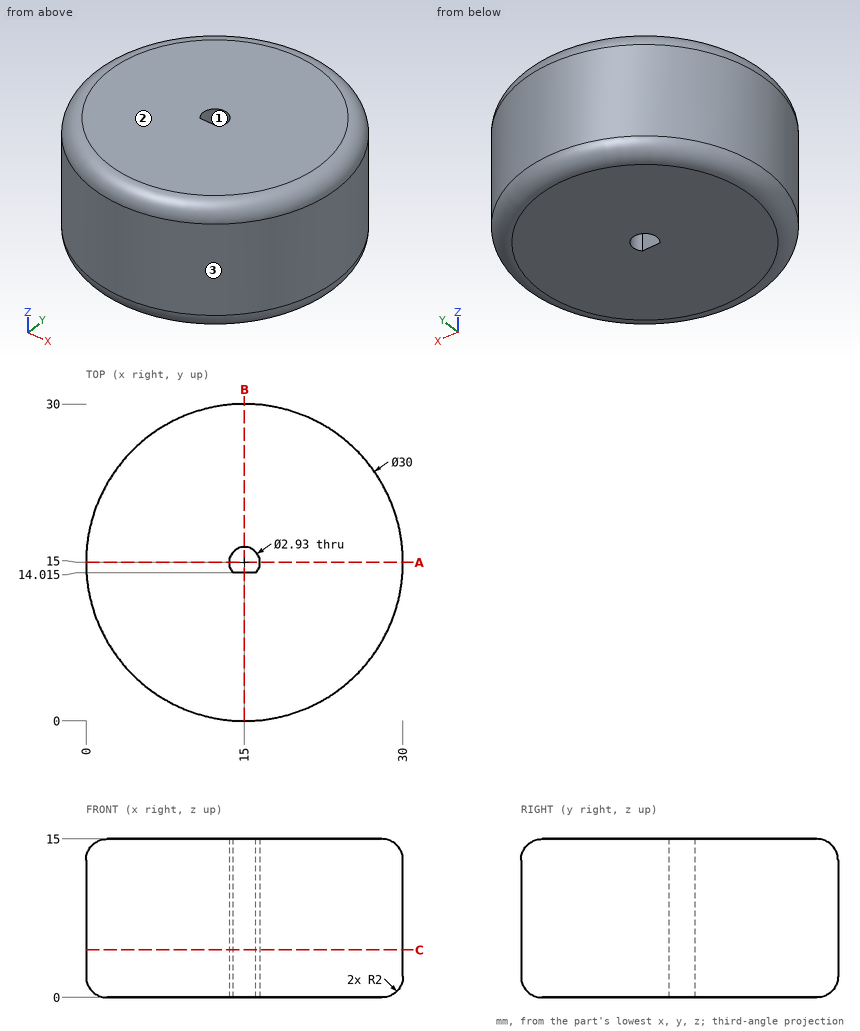
Study the drawing (mm; zero at the part's minimum x, y, z) and answer. Give positions to 0.01 mm unless a question says otherwise; leave off trailing zeros. Loops run counter-clockwise (first coordinate to the right, second up) from the corner with the lowest first, then second, coordinate; pieces in that order, holes last. Notation, with made-up numbers: (31.5, 75.5) - (41.5, 75.5) arc R27 ccw to (41.5, 99.5) - close; hole circle Ø10 at (-34.5, 9.25). An arc over 180 degrees is marked (long way). Use CSV: the item, a comma, the result in double quotes. Start each with the question number.
(1) Find section B-B, the plane x = 15. Determine the outline of the cut face in (y, z) (3 decimals), plus the area to 3 significant figures.
(2) Each of these flat-tipped pins is pushed along its axis until it touches: pin 1 (6 mm diameter, centred on y = 19, z = 11, fed in from -X); pin 2 (1 mm diameter, centred on y = 13, z = 9, fed in from +X); pin 3 (1.5 mm diameter, centred on y = 9.5, z = 11, fed in from +X); pin 4 (1.8 mm diameter, centred on x = 15, y = 15, fed in from -Z). Where does it stop, or does it pass through?
(3) Find section C-C, the plane z = 4.5. Determine the outline of the cut face in (x, y) (1 decimal), plus the area to 3 significant figures.
(4) Find section A-A, the plane y = 15. Determine the outline of the cut face in (x, z) (3 decimals), plus the area to 3 significant figures.
(5) Determine the mould class of the marked faces 1, 2 and 3 for opening direction Y: released by +Y, released by -Y, zero draft, split by the parting line, or undercut.
(6) Find the intervals of material crossed by L1, parallel to Y at x = 15, z = 7 (3 decimals); L2, parallel to Z at x = 25, y = 25.5; L3, parallel to Y at x = 28, z = 7.5, in increasing order.
Results found:
1,outline,"(0, 2) arc R2 ccw to (2, 0) - (14.015, 0) - (14.015, 15) - (2, 15) arc R2 ccw to (0, 13) - close; (16.465, 0) - (28, 0) arc R2 ccw to (30, 2) - (30, 13) arc R2 ccw to (28, 15) - (16.465, 15) - close"
1,area,"410 mm^2"
2,pin 1,"x = 0.03"
2,pin 2,"x = 29.92"
2,pin 3,"x = 29.23"
2,pin 4,"through"
3,outline,"circle Ø30 at (15, 15); hole (13.9, 14) - (16.1, 14) arc R1.5 ccw (long way) to start"
3,area,"701 mm^2"
4,outline,"(0, 2) arc R2 ccw to (2, 0) - (13.535, 0) - (13.535, 15) - (2, 15) arc R2 ccw to (0, 13) - close; (16.465, 0) - (28, 0) arc R2 ccw to (30, 2) - (30, 13) arc R2 ccw to (28, 15) - (16.465, 15) - close"
4,area,"403 mm^2"
5,face 1,"undercut"
5,face 2,"zero draft"
5,face 3,"split by the parting line"
6,L1,"0 to 14.015, 16.465 to 30"
6,L2,"0.68 to 14.32"
6,L3,"7.52 to 22.48"
